Input: dimensioned drawing with shaded views. Units: mm. Origin: part minimum x, y, z. A direction names the side the tool comes from. Round coordinates to 2 decimals unless told otherwise and drop trailing zeros. Write each loop counter-clockwise with the first axis right and the second up, starting at its lowest first coordinate (ties: lowest second). Pieces come first, ordered by that corner, then holes. Notation, with made-up numbers: M 21.5,-15.75 L 50.5,-15.75 A32 cw 50.5,10.25 Z; hole C 2,18.5 d11. An arc over 180 degrees is marked long. Put each result on its own line as item: value. Start each with the question number.
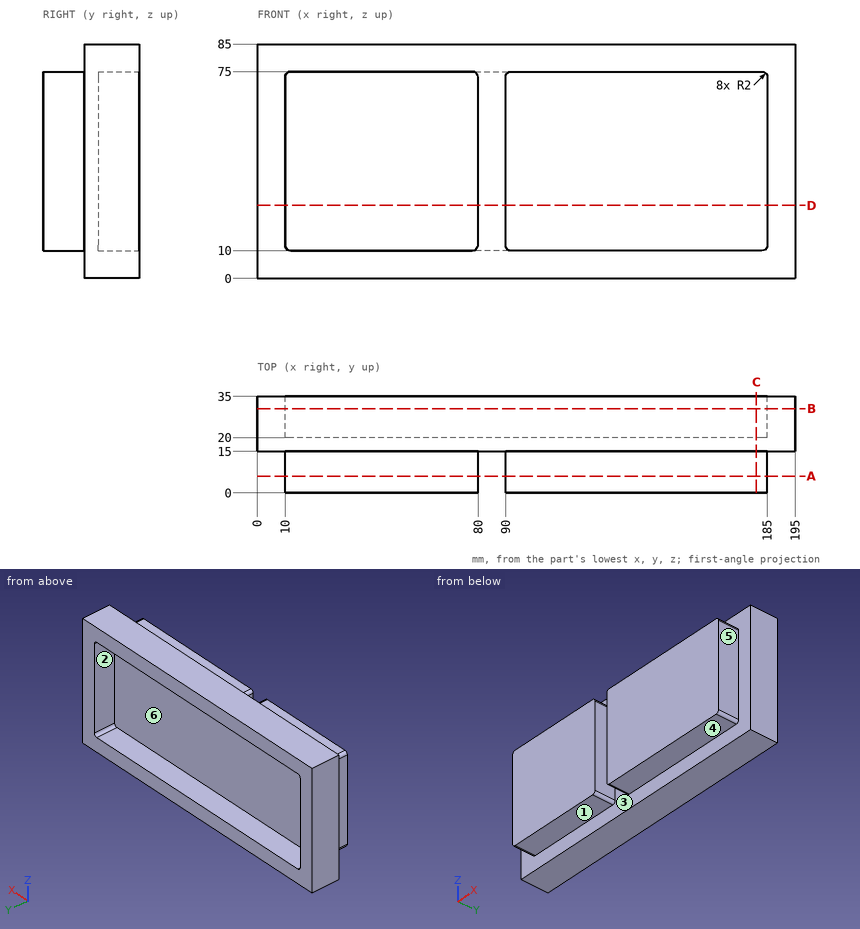
1) Access query for the marked faces 1, 2 and 3. Directions: +Z, -Z, +X, -X, +Y, -Y. A direction counts if a zero-diameter tool reaches every point of the face in a straight line with its end or side. Return the directions, or none.
2) Section A-A, the plane y = 6. Output: boundary loops of the cut face in (x, z), and give its area (3 significant figures).
3) Section C-C, the plane x = 181. Output: boundary loops of the cut face in (y, z), and give its area (3 significant figures).
4) Section D-D, the plane z = 26.5. Output: boundary loops of the cut face in (x, y), and give its area (3 significant figures).
5) Ray query, probe 1 along X at (y, z) = (14, 18); probe 2 along X at (y, z) = (30.5, 32); probe 3 along Z at (x, y) = (182, 29.5). Return the intervals inside material, ascending.
6) Draft query along Z for the marked faces 4, 5 and 6. Return one class per face: +Z half, -Z half, draft (parallel to the pull), parting line (faces both ways), or undercut.
7) First-contact query: pin 1 (7.5 mm diameter, centred on y = 5.5, z = 54.5, fed in from +X); pin 2 (12 mm diameter, centred on x = 58, y = 4.5, fed in from +Z); pin 3 (7.5 mm diameter, centred on y = 10, z = 48, fed in from -X). Flat tips, straight axial feed; report the tip coordinate or a pass-through.
8) Section B-B, the plane y = 30.5. Output: boundary loops of the cut face in (x, z).
Solved:
1. face 1: -Z, +X, -X, -Y
1. face 2: +Y
1. face 3: -Y
2. outline: M 10,12 A2 ccw 12,10 L 78,10 A2 ccw 80,12 L 80,73 A2 ccw 78,75 L 12,75 A2 ccw 10,73 Z; M 90,12 A2 ccw 92,10 L 183,10 A2 ccw 185,12 L 185,73 A2 ccw 183,75 L 92,75 A2 ccw 90,73 Z
2. area: 10,700 mm2
3. outline: M 0,10 L 15,10 L 15,0 L 35,0 L 35,10 L 20,10 L 20,75 L 35,75 L 35,85 L 15,85 L 15,75 L 0,75 Z
3. area: 1,700 mm2
4. outline: M 0,15 L 10,15 L 10,0 L 80,0 L 80,15 L 90,15 L 90,0 L 185,0 L 185,15 L 195,15 L 195,35 L 185,35 L 185,20 L 10,20 L 10,35 L 0,35 Z
4. area: 3,750 mm2
5. probe 1: x = 10 to 80, 90 to 185
5. probe 2: x = 0 to 10, 185 to 195
5. probe 3: z = 0 to 10, 75 to 85
6. face 4: -Z half
6. face 5: draft
6. face 6: undercut
7. pin 1: stops at x = 185
7. pin 2: stops at z = 75
7. pin 3: stops at x = 10
8. outline: M 0,0 L 195,0 L 195,85 L 0,85 Z; hole M 10,12 A2 ccw 12,10 L 183,10 A2 ccw 185,12 L 185,73 A2 ccw 183,75 L 12,75 A2 ccw 10,73 Z
